from build123d import *

# Parameters (mm, degrees)
M10X1_52_D            = 8.5
M10X1_52_DEPTH        = 37.5
M10X1_52_CSINK_D      = 11
M10X1_52_CSINK_ANGLE  = 90
M10X1_52_TIP          = 2.553657631
HOLE_WIZARD_M81_D     = 6.8
HOLE_WIZARD_M81_DEPTH = 30
HOLE_WIZARD_M81_TIP   = 2.042926105
SKETCH_6_W            = 2.5
SKETCH_6_H            = 1.1
CHAMFER_1_SIZE        = 2
CHAMFER_2_SIZE        = 1
CHAMFER_3_SIZE        = 2.2
FILLET_1_R            = 1


with BuildPart() as part:
    # Эскиз1 → Повернуть1 (revolve)
    with BuildSketch(Plane.XY, mode=Mode.PRIVATE) as revolve_1_sk:
        Polygon((0, 0), (0, 13), (30, 13), (30, 17.5), (40, 17.5), (40, 13), (90, 13), (90, 10), (124, 10), (124, 8), (140, 8), (140, 0), align=None)
    revolve(revolve_1_sk.sketch.rotate(Axis((-123.335902371, 0, 0), (1, 0, 0)), 90), axis=Axis((-123.335902371, 0, 0), (1, 0, 0)))

    # Отверстие обработанное метчиком M10x1.52
    with Locations(Plane.ZY):
        with Locations((0, 0)):
            CounterSinkHole(M10X1_52_D / 2, M10X1_52_CSINK_D / 2, depth=M10X1_52_DEPTH, counter_sink_angle=M10X1_52_CSINK_ANGLE)
            with Locations((0, 0, -(M10X1_52_DEPTH + M10X1_52_TIP / 2))):  # 118° drill point
                Cone(0, M10X1_52_D / 2, M10X1_52_TIP, mode=Mode.SUBTRACT)

    # Отверстие обработанное метчиком M81
    with Locations(Plane(origin=(140, 0, 0), x_dir=(0, 0, -1), z_dir=(1, 0, 0))):
        with Locations((0, 0)):
            Hole(HOLE_WIZARD_M81_D / 2, depth=HOLE_WIZARD_M81_DEPTH)
            with Locations((0, 0, -(HOLE_WIZARD_M81_DEPTH + HOLE_WIZARD_M81_TIP / 2))):  # 118° drill point
                Cone(0, HOLE_WIZARD_M81_D / 2, HOLE_WIZARD_M81_TIP, mode=Mode.SUBTRACT)

    # Эскиз6 → Вырез-Повернуть1 (revolve, cut)
    with BuildSketch(Plane.XY, mode=Mode.PRIVATE) as cut_revolve_1_sk:
        with Locations((125.25, 7.45)):
            Rectangle(SKETCH_6_W, SKETCH_6_H)
    revolve(cut_revolve_1_sk.sketch.rotate(Axis((0, 0, 0), (1, 0, 0)), 90), axis=Axis((0, 0, 0), (1, 0, 0)), mode=Mode.SUBTRACT)

    # Фаска1
    chamfer_1_edges = [part.edges().sort_by_distance(p)[0] for p in [
        (0, 0, -13),
        (140, 0, -8),
    ]]
    chamfer(chamfer_1_edges, length=CHAMFER_1_SIZE)

    # Фаска2
    chamfer_2_edges = [part.edges().sort_by_distance(p)[0] for p in [
        (90, 0, -13),
    ]]
    chamfer(chamfer_2_edges, length=CHAMFER_2_SIZE)

    # Фаска3
    # the kernel refuses this chamfer: 2.2 mm, written as the material it takes off along each edge
    with BuildSketch(Plane(origin=(126.5, 0, 0), x_dir=(0, 0, 1), z_dir=(0, 1, 0))) as chamfer_3_piece_1_section:
        Polygon((8 - CHAMFER_3_SIZE, 0), (8, CHAMFER_3_SIZE), (8, 0), align=None)
    chamfer_3_piece_1 = revolve(axis=Axis((126.5, 0, 0), (1, 0, 0)), mode=Mode.PRIVATE)
    chamfer_3_piece_1 = chamfer_3_piece_1 - Plane(origin=(128.148983784, 0, 0), x_dir=(0, 0, 1), z_dir=(-1, 0, 0)) * Cylinder(6.9, 32, mode=Mode.PRIVATE)
    add(chamfer_3_piece_1, mode=Mode.SUBTRACT)

    # Скругление1
    fillet_1_edges = [part.edges().sort_by_distance(p)[0] for p in [
        (124, 0, -6.9),
    ]]
    fillet(fillet_1_edges, radius=FILLET_1_R)


solid = part.part
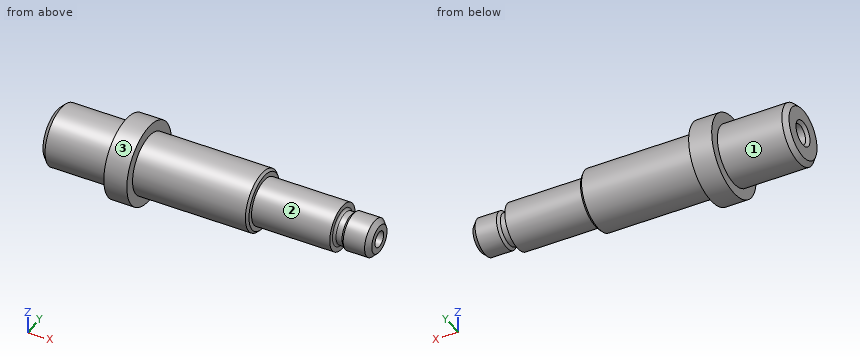
CAD build for the part. Positions are in the model's coordinates, mm. Face numbers are marked on the shaded views. A direction names the side the tool comes from. Give positions to 0.01 mm unless a question says otherwise; leave off trailing zeros. Loops run counter-clockwise (first coordinate to the right, second up) from the corner with the lowest first, then second, coordinate; pieces in that order, holes last. Notation, with made-up numbers: M -36.5,15.25 L 19.5,15.25 A19 ccw 19.5,21.25 Z; hole C 16,-24.75 d1. An arc over 180 degrees is marked long. Answer in a Markdown table with one row per item. Add a question column.
Item 1: Band-saw the part on B-B on z = 15. Give the cut face in (x, y), then the cut area to 3 significant figures.
Item 2: Band-saw the part on A-A on x = 80.5. Give the cut face in (y, z).
Item 3: Probe probe 1 along Y at (x, z) = (123.5, 0); probe 2 along Y at (x, z) = (130, 0). List the from-to ranges inside material, lowest first.
Item 4: Drop flat-ended pins along their axis: P1, Ø6, axis at y = 0, z = 0, coming from the +X side; P2, Ø1, axis at x = 126, y = -1.5, coming from the +Z side; P3, Ø6, axis at x = 78.5, z = 11.5, coming from the +Y side. Give the stop position or say it passes through.
Item 5: Tool access for the marked faces 1, 2 and 3: list every direction of +Z, -Z, +X, -X, +Y, -Y with a clear straight run to the whole face (end or side of a thin tool).
Reply:
| question | item | result |
|---|---|---|
| 1 | outline | M 30,-9.01 L 40,-9.01 L 40,9.01 L 30,9.01 Z |
| 1 | area | 180 mm^2 |
| 2 | outline | C 0,0 d26 |
| 3 | probe 1 | y = -10 to -3.4, 3.4 to 10 |
| 3 | probe 2 | y = -8 to -3.4, 3.4 to 8 |
| 4 | P1 | stops at x = 109.76 |
| 4 | P2 | stops at z = 6.83 |
| 4 | P3 | stops at y = 9.84 |
| 5 | face 1 | -X |
| 5 | face 2 | +X |
| 5 | face 3 | +X, -X |
